Design review of the part built by this model. Coordinates are the model's own, in mm. A direction names the side the tool comes from. Coordinates: 2 decimals unless noted, no trailing zeros. Loops run counter-clockwise (first coordinate to the right, second up) from the corner with the lowest first, then second, coordinate; pieces in that order, holes last.
Q1. Add section C-C on x = -8. Give the boundary of the cut face in (y, z), and give its area (3 significant figures).
Q2. Add section A-A on y = 24. Give the boundary of the cut face in (x, z).
Q3. Add section B-B on x = -5. Give the boundary of the cut face in (y, z).
Q4. Draft analysis for pull direction X (two halves, no side actions). For faces 4 (the face through (-5.195, -25.487, 9.014)), 5 (the face through (0, -24, 8)), 6 (the face through (-10, 0, 18)), 7 (the face through (4.805, 25.487, 8.986)), state which applies: released by +X, released by -X, zero draft, split by the parting line, or undercut.
Q5. Machinability: for faces 1 (the face through (0, 20, 23)), 2 (the face through (0, -20, 4)), 3 (the face through (0, -20, 23)), which of the approach directions +Z, -Z, +X, -X, +Y, -Y give a long, thin tool a straight path to every point of the face, cutting with its end or side? Answer none if there is none.
Q6. For P1, Ø6.5, axis at x = 2.5, y = -23, coming from the -Z side; P2, Ø2, axis at x = -1, z = 28.5, coming from the -Y side; P3, Ø3.5, axis at x = 5, y = -24, coming from the +Z side, all flat-tipped, find the tip position at first contact; note any pin that passes through.
Q7. Add section D-D on z = 6. Give the boundary of the cut face in (x, y).
Q8. Wall thickness on probe 1 along Y at (x, z) = (5, 8.7); probe 2 along Y at (x, z) = (8.5, 14); probe 3 along Z at (x, y) = (-9, -1): over which ranges is each line inside the solid? List them lowest first.
```python
from build123d import *

# Parameters (mm, degrees)
SKETCH1_W           = 20
SKETCH1_H           = 40
BOSS_EXTRUDE1_DEPTH = 37
SKETCH2_W           = 20
SKETCH2_H           = 2
BOSS_EXTRUDE2_DEPTH = 8
SKETCH3_R           = 1.5
CUT_EXTRUDE2_DEPTH  = 48.465777145
SKETCH4_R           = 2.5
BOSS_EXTRUDE3_DEPTH = 8


with BuildPart() as part:
    # Sketch1 → Boss-Extrude1 (new body)
    with BuildSketch(Plane.XY):
        Rectangle(SKETCH1_W, SKETCH1_H)
    extrude(amount=BOSS_EXTRUDE1_DEPTH)

    # Sketch2 → Boss-Extrude2 (add)
    with BuildSketch(Plane(origin=(0, 20, 0), x_dir=(1, 0, 0), z_dir=(0, 1, 0))):
        with Locations((0, -9)):
            Rectangle(SKETCH2_W, SKETCH2_H)
    boss_extrude2 = extrude(amount=BOSS_EXTRUDE2_DEPTH)

    # Sketch3 → Cut-Extrude2 (cut, symmetric)
    with BuildSketch(Plane.XY):
        with Locations((5, 24)):
            Circle(SKETCH3_R)
        with Locations((-5, 24)):
            Circle(SKETCH3_R)
    cut_extrude2 = extrude(amount=CUT_EXTRUDE2_DEPTH, both=True, mode=Mode.SUBTRACT)

    # Mirror3: Boss-Extrude2, Cut-Extrude2 across plane
    add(boss_extrude2.mirror(Plane.ZX))
    add(cut_extrude2.mirror(Plane.ZX), mode=Mode.SUBTRACT)

    # Sketch4 → Boss-Extrude3 (add)
    with BuildSketch(Plane(origin=(0, 0, 0), x_dir=(-1, 0, 0), z_dir=(0, 0, -1))):
        with Locations((0, -12)):
            Circle(SKETCH4_R)
    extrude(amount=BOSS_EXTRUDE3_DEPTH)


solid = part.part
```
Entries:
1. outline: (-28, 8) - (-20, 8) - (-20, 0) - (20, 0) - (20, 8) - (28, 8) - (28, 10) - (20, 10) - (20, 37) - (-20, 37) - (-20, 10) - (-28, 10) - close
1. area: 1,510 mm2
2. outline: (-10, 8) - (-6.5, 8) - (-6.5, 10) - (-10, 10) - close; (-3.5, 8) - (3.5, 8) - (3.5, 10) - (-3.5, 10) - close; (6.5, 8) - (10, 8) - (10, 10) - (6.5, 10) - close
3. outline: (-28, 8) - (-25.5, 8) - (-25.5, 10) - (-28, 10) - close; (-22.5, 8) - (-20, 8) - (-20, 0) - (20, 0) - (20, 8) - (22.5, 8) - (22.5, 10) - (20, 10) - (20, 37) - (-20, 37) - (-20, 10) - (-22.5, 10) - close; (25.5, 8) - (28, 8) - (28, 10) - (25.5, 10) - close
4. face 4: undercut
4. face 5: zero draft
4. face 6: released by -X
4. face 7: undercut
5. face 1: +Z, +X, -X, +Y
5. face 2: -Z, +X, -X, -Y
5. face 3: +Z, +X, -X, -Y
6. P1: stops at z = 0
6. P2: stops at y = -20
6. P3: stops at z = 10
7. outline: (-10, -20) - (10, -20) - (10, 20) - (-10, 20) - close
8. probe 1: y = -28 to -25.5, -22.5 to 22.5, 25.5 to 28
8. probe 2: y = -20 to 20
8. probe 3: z = 0 to 37
